Work out the finished part from the listing and answer in its coordinate system (mm). A direction names the side the tool comes from. Give positions to 0.01 mm unless a question says otherwise; leave off trailing zeros. Write each loop counter-clockwise with the first axis right and the second up, starting at its lowest first coordinate (ties: lowest second). Pieces come first, ordered by that corner, then holes. Notation, with made-up numbers: (-21.5, 53.5) -> (-6.5, 53.5) arc R11 ccw to (-6.5, 72.5) -> close; hole circle Ø3 at (52.5, 59). An arc over 180 degrees is marked (long way). Use a Markdown table: item, result. Add a question column.
Q1. Consider line 1 (Z direction, x = 0, y = -92); line 2 (Z direction, x = 0, y = -302); line 3 (Y direction, x = 93, z = 7.5). Determine where each line is inside the solid, lowest interval first.
Q2. Each of these flat-tipped pins is pushed along its axis until it touches: pin 1 Ø6 at (y, z) = (-81.5, 88.5) entering from -X; pin 2 Ø5 at (x, y) = (-84.5, -208.5) entering from +Z; pin 3 Ø5 at (x, y) = (-65, -96.5) entering from -Z; pin 4 Ø6 at (x, z) = (-90, -100) entering from +Y. Where does it stop, or does it pass through?
Q3. Section C-C, the plane y = -238 is taken. Give the vertices of the cut face in (x, z), plus the area to 3 significant figures.
Q4. Section B-B, the plane y = -205.5 is taken. Give the vertices of the cut face in (x, z), plus the area to 3 significant figures.
Q5. For a pull along Z with two mould halves and no side action, classify faces 1 (the face through (-4.88, -306.41, 37.18)), 2 (the face through (26, -297, -26)), 3 (the face through (-17, 0, -15)) as pulls with the +Z half, pulls with the -Z half, needs draft (parallel to the pull), parting line crosses it, or undercut.
Q6. Section A-A, the plane y = -72 is taken. Give the vertices of the cut face in (x, z), plus the area to 3 significant figures.
Q7. For faces 4 (the face through (32.907, -304.888, 10.363)), 5 (the face through (-23, -16, 76)), 6 (the face through (116.452, -243.858, 119.617)), determine the directions among +Z, -Z, +X, -X, +Y, -Y from which every point of the face is accessible in a straight line to the end or side of a thin tool.
from build123d import *

# Parameters (mm, degrees)
F0_R      = 130
F1_DEPTH  = 300
F2_R      = 37.5
F3_DEPTH  = 13
F4_R      = 117
F4_R_2    = 72
F5_DEPTH  = 13
F5_TAPER  = 30
F6_R      = 22.5
F7_DEPTH  = 7
F7_TAPER  = 30
F8_T      = -3
F10_START = 25
F9_R      = 45
F10_DEPTH = 135


with BuildPart() as f1:
    # F0 (on Front) → F1 (new body)
    with BuildSketch(Plane.XZ):
        Circle(F0_R)
    extrude(amount=F1_DEPTH)

    # F2 (on face) → F3 (join)
    with BuildSketch(Plane.XZ.offset(300)):
        Circle(F2_R)
    extrude(amount=F3_DEPTH)

    # F4 (on face) → F5 (cut)
    with BuildSketch(Plane(origin=(0, 0, 0), x_dir=(-1, 0, 0), z_dir=(0, 1, 0))):
        Circle(F4_R)
        Circle(F4_R_2, mode=Mode.SUBTRACT)
    extrude(amount=-F5_DEPTH, taper=F5_TAPER, mode=Mode.SUBTRACT)

    # F6 (on face) → F7 (join)
    with BuildSketch(Plane(origin=(0, 0, 0), x_dir=(-1, 0, 0), z_dir=(0, 1, 0))):
        Circle(F6_R)
    extrude(amount=F7_DEPTH, taper=F7_TAPER)

    # F8
    f8_openings = [f1.faces().sort_by_distance(p)[0] for p in [
        (0, -313, 0),
    ]]
    offset(amount=F8_T, openings=f8_openings, kind=Kind.INTERSECTION)

    # F9 (on Right) → F10 (join)
    with BuildSketch(Plane.YZ.offset(F10_START)):
        with Locations((-238, 75)):
            Circle(F9_R)
    extrude(amount=F10_DEPTH)


solid = f1.part
Result set:
| question | item | result |
|---|---|---|
| 1 | line 1 | z = -130 to -127, 127 to 130 |
| 1 | line 2 | z = -37.5 to -34.5, 34.5 to 37.5 |
| 1 | line 3 | y = -300 to -297, -16 to -13 |
| 2 | pin 1 | stops at x = -97.93 |
| 2 | pin 2 | stops at z = 100.88 |
| 2 | pin 3 | stops at z = -113.99 |
| 2 | pin 4 | passes through |
| 3 | outline | (50, 120) arc R130 ccw (long way) to (126.49, 30) -> (160, 30) -> (160, 120) -> close; hole (25, 30) -> (25, 120) -> (41.58, 120) arc R127 ccw (long way) to (123.41, 30) -> close |
| 3 | area | 14,200 mm2 |
| 4 | outline | (75.08, 106.12) arc R130 ccw (long way) to (122.37, 43.88) -> (160, 43.88) -> (160, 106.12) -> close; hole (25, 43.88) -> (25, 106.12) -> (69.76, 106.12) arc R127 ccw (long way) to (119.18, 43.88) -> close |
| 4 | area | 10,600 mm2 |
| 5 | face 1 | parting line crosses it |
| 5 | face 2 | undercut |
| 5 | face 3 | needs draft |
| 6 | outline | circle Ø260 at (0, 0); hole circle Ø254 at (0, 0) |
| 6 | area | 2,420 mm2 |
| 7 | face 4 | -Y |
| 7 | face 5 | none |
| 7 | face 6 | +X |
